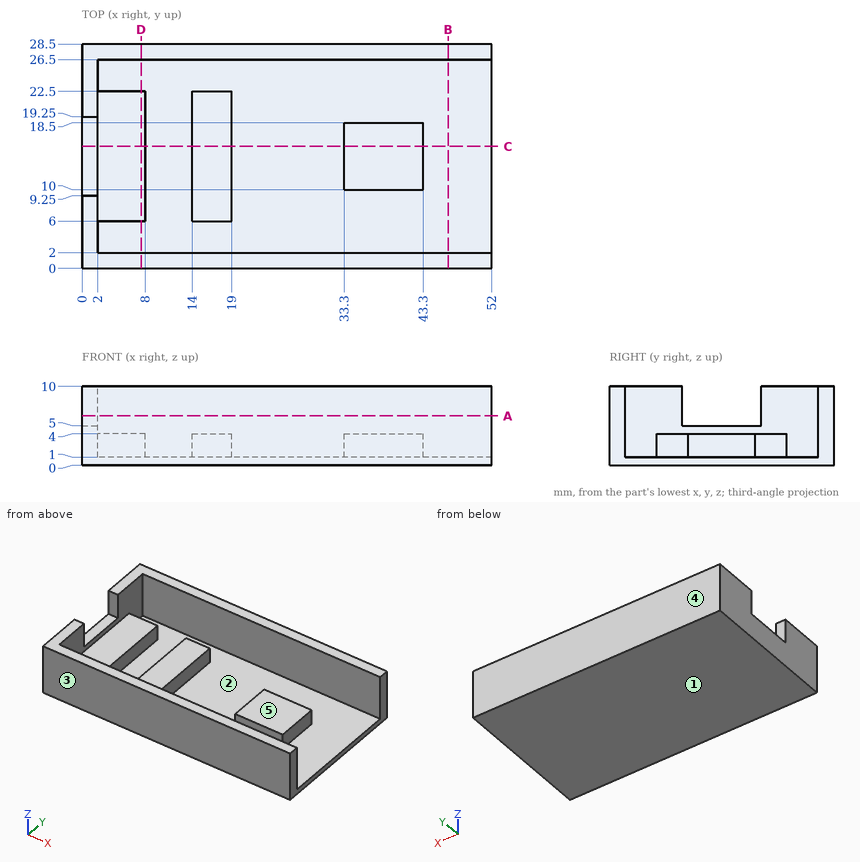
Geometry check sheet. Reference: drawing and pictorial views, mm from the part's lowest x, y, z. A direction names the side the tool comes from. Give positions to 0.01 mm unless a question says otherwise; leave off trailing zeros. Order: outer loops, then holes, each group sorted by start corner. A loop starts at its lowest first (then second) coordinate and runs counter-clockwise, first axis right, second up. Notation, with made-up numbers: M -12,16 L 17,16 A27 ccw 17,53 Z; hole C -22.75,-14 d9. An arc over 180 degrees is marked long. Answer in a Markdown table with one row per item. Add a question column.
Q1. Thickness scan on L1, parallel to X at y = 15, z = 1.25; L2, parallel to Y at x = 28, z = 9; L3, parallel to X at y = 21.25, z = 2. Record the ranges inside material, lowest first.
Q2. Sectioned sample at D-D, the plane x = 7.5. Record the boundary of the cut face in (y, z), and give its area (3 significant figures).
Q3. Sectioned sample at A-A, the plane z = 6.25. Record the boundary of the cut face in (x, y), and give its area (3 significant figures).
Q4. Sectioned sample at C-C, the plane y = 15.5. Record the boundary of the cut face in (x, z), and give its area (3 significant figures).
Q5. Sectioned sample at B-B, the plane x = 46.5. Record the boundary of the cut face in (y, z), and give its area (3 significant figures).
Q6. Access from +Z, -Z, +X, -X, +Y, -Y to the whole of each face (thin tool, end or side, straight path). Record for the marked faces 4 and 5.
Q7. Release check for a two-part mould opening along Y. For the marked faces 1, 2 and 3 record: released by +Y, released by -Y, zero draft, split by the parting line, or undercut.
Q8. Gauge pin test, flat ends, axial feed: pin 1 Ø5 at (y, z) = (3.5, 1.5) entering from -X; pin 2 Ø9.5 at (x, y) = (39.5, 14.5) entering from +Z; pin 3 Ø0.9 at (y, z) = (12.5, 3) entering from +X; pin 4 Ø5 at (x, y) = (32.5, 6) entering from +Z. Record the tip position at first contact, or that the pin passes through.
Verdict:
| question | item | result |
|---|---|---|
| 1 | L1 | 0 to 8, 14 to 19, 33.3 to 43.3 |
| 1 | L2 | 0 to 2, 26.5 to 28.5 |
| 1 | L3 | 0 to 8, 14 to 19 |
| 2 | outline | M 0,0 L 28.5,0 L 28.5,10 L 26.5,10 L 26.5,1 L 22.5,1 L 22.5,4 L 6,4 L 6,1 L 2,1 L 2,10 L 0,10 Z |
| 2 | area | 114 mm² |
| 3 | outline | M 0,0 L 52,0 L 52,2 L 2,2 L 2,9.25 L 0,9.25 Z; M 0,19.25 L 2,19.25 L 2,26.5 L 52,26.5 L 52,28.5 L 0,28.5 Z |
| 3 | area | 237 mm² |
| 4 | outline | M 0,0 L 52,0 L 52,1 L 43.3,1 L 43.3,4 L 33.3,4 L 33.3,1 L 19,1 L 19,4 L 14,4 L 14,1 L 8,1 L 8,4 L 2,4 L 2,5 L 0,5 Z |
| 4 | area | 123 mm² |
| 5 | outline | M 0,0 L 28.5,0 L 28.5,10 L 26.5,10 L 26.5,1 L 2,1 L 2,10 L 0,10 Z |
| 5 | area | 64.5 mm² |
| 6 | face 4 | +Z, -Z, +X, -X, +Y |
| 6 | face 5 | +Z, +X |
| 7 | face 1 | zero draft |
| 7 | face 2 | undercut |
| 7 | face 3 | released by -Y |
| 8 | pin 1 | x = 0 |
| 8 | pin 2 | z = 4 |
| 8 | pin 3 | x = 43.3 |
| 8 | pin 4 | z = 1 |
